The model under review builds one solid part; all positions refer to its coordinate system, in mm. A direction names the side the tool comes from. Give positions to 0.01 mm unless a question says otherwise; leave off trailing zeros. Write each loop counter-clockwise with the first axis right and the second up, starting at its lowest first coordinate (ties: lowest second). Pieces come first, ordered by that corner, then holes. Notation, with made-up numbers: M -38,-15 L -4,-15 A21 ccw -4,16 Z; hole C -20.75,62.25 d1. An arc over 180 degrees is marked long. Write item = value, one per line. Start each with the question number.
```python
from build123d import *

# Parameters (mm, degrees)
SKETCH_1_W          = 15
SKETCH_1_H          = 15
SKETCH_1_W_2        = 12
SKETCH_1_H_2        = 12
EXTRUDE_1_DEPTH     = 600
SKETCH_2_R          = 2.25
CUT_EXTRUDE_1_DEPTH = 25
SKETCH_3_R          = 2.25
CUT_EXTRUDE_2_DEPTH = 25
SKETCH_4_R          = 5
CUT_EXTRUDE_3_DEPTH = 10
SKETCH_5_R          = 5
CUT_EXTRUDE_4_DEPTH = 10
SKETCH_6_R          = 2.7
CUT_EXTRUDE_5_DEPTH = 20
SKETCH_7_R          = 5
CUT_EXTRUDE_6_DEPTH = 3


with BuildPart() as part:
    # ｽｹｯﾁ1 → ﾎﾞｽ - 押し出し1 (new body)
    with BuildSketch(Plane.XY):
        Rectangle(SKETCH_1_W, SKETCH_1_H)
        Rectangle(SKETCH_1_W_2, SKETCH_1_H_2, mode=Mode.SUBTRACT)
    extrude(amount=EXTRUDE_1_DEPTH)

    # ｽｹｯﾁ2 → ｶｯﾄ - 押し出し1 (cut)
    with BuildSketch(Plane(origin=(7.5, 0, 0), x_dir=(0, 0, -1), z_dir=(1, 0, 0))):
        with Locations((-592.5, 0)):
            Circle(SKETCH_2_R)
        with Locations((-7.5, 0)):
            Circle(SKETCH_2_R)
        with Locations((-336.5, 0)):
            Circle(SKETCH_2_R)
        with Locations((-263.5, 0)):
            Circle(SKETCH_2_R)
    extrude(amount=-CUT_EXTRUDE_1_DEPTH, mode=Mode.SUBTRACT)

    # ｽｹｯﾁ3 → ｶｯﾄ - 押し出し2 (cut)
    with BuildSketch(Plane(origin=(0, 7.5, 0), x_dir=(1, 0, 0), z_dir=(0, 1, 0))):
        with Locations((0, -22.5)):
            Circle(SKETCH_3_R)
        with Locations((0, -577.5)):
            Circle(SKETCH_3_R)
        with Locations((0, -351.5)):
            Circle(SKETCH_3_R)
        with Locations((0, -248.5)):
            Circle(SKETCH_3_R)
    extrude(amount=-CUT_EXTRUDE_2_DEPTH, mode=Mode.SUBTRACT)

    # ｽｹｯﾁ4 → ｶｯﾄ - 押し出し3 (cut)
    with BuildSketch(Plane(origin=(0, 7.5, 0), x_dir=(1, 0, 0), z_dir=(0, 1, 0))):
        with Locations((0, -577.5)):
            Circle(SKETCH_4_R)
        with Locations((0, -351.5)):
            Circle(SKETCH_4_R)
        with Locations((0, -248.5)):
            Circle(SKETCH_4_R)
        with Locations((0, -22.5)):
            Circle(SKETCH_4_R)
    extrude(amount=-CUT_EXTRUDE_3_DEPTH, mode=Mode.SUBTRACT)

    # ｽｹｯﾁ5 → ｶｯﾄ - 押し出し4 (cut)
    with BuildSketch(Plane(origin=(7.5, 0, 0), x_dir=(0, 0, -1), z_dir=(1, 0, 0))):
        with Locations((-592.5, 0)):
            Circle(SKETCH_5_R)
        with Locations((-336.5, 0)):
            Circle(SKETCH_5_R)
        with Locations((-263.5, 0)):
            Circle(SKETCH_5_R)
        with Locations((-7.5, 0)):
            Circle(SKETCH_5_R)
    extrude(amount=-CUT_EXTRUDE_4_DEPTH, mode=Mode.SUBTRACT)

    # ｽｹｯﾁ6 → ｶｯﾄ - 押し出し5 (cut)
    with BuildSketch(Plane(origin=(7.5, 0, 0), x_dir=(0, 0, -1), z_dir=(1, 0, 0))):
        with Locations((-480, 0)):
            Circle(SKETCH_6_R)
        with Locations((-443, 0)):
            Circle(SKETCH_6_R)
        with Locations((-157, 0)):
            Circle(SKETCH_6_R)
        with Locations((-120, 0)):
            Circle(SKETCH_6_R)
    extrude(amount=-CUT_EXTRUDE_5_DEPTH, mode=Mode.SUBTRACT)

    # ｽｹｯﾁ7 → ｶｯﾄ - 押し出し6 (cut)
    with BuildSketch(Plane.ZY.offset(7.5)):
        with Locations((120, 0)):
            Circle(SKETCH_7_R)
        with Locations((157, 0)):
            Circle(SKETCH_7_R)
        with Locations((443, 0)):
            Circle(SKETCH_7_R)
        with Locations((480, 0)):
            Circle(SKETCH_7_R)
    extrude(amount=-CUT_EXTRUDE_6_DEPTH, mode=Mode.SUBTRACT)


solid = part.part
```
Item 1: For faces 4 (the cylindrical face through (6.76, -1.915, 587.881)), 5 (the cylindrical face through (-1.08, 6.76, 27.38)), 6 (the cylindrical face through (-6.76, 1.5, 447.77)), 7 (the flat face through (7.5, 0, 296)), 8 (the flat face through (0, -6, 296)), list the 3-axis set-ups (+Z, -Z, +X, -X, +Y, -Y) from which the entire face can be reached by the end or side of a thin tool; tool diameter is ignored.
Item 2: To check wall thickness, follow probe 1 along Z at (x, y) = (0, 6.6); probe 2 along X at (y, z) = (7, 351.5); probe 3 along Y at (x, z) = (4.5, 437). State the ranges of each line that lie inside material, in increasing order. Write a range as [from, to].
Item 3: We need section A-A, the plane z = 228. Write out the cut boundary in (x, y), and give its area (3 significant figures).
Item 4: Clearance check with flat-ended pins moving along their axes: P1, Ø4.5, axis at y = 0, z = 480, coming from the -X side; P2, Ø6, axis at y = 0, z = 336.5, coming from the +X side; P3, Ø6, axis at x = 0, z = 22.5, coming from the +Y side; P4, Ø7, axis at y = 0, z = 157, coming from the -X side. State where each tip first meets the part, or that it passes through.
Item 5: The part is to be moulded in two halves that separate along Z. For faces 1 (the cylindrical face through (6.76, 1.5, 331.73)), 2 (the flat face through (-6, 0, 296)), 3 (the flat face through (-7, 0, 600)), say which applies: released by +Z, released by -Z, zero draft, split by the parting line, or undercut.
Worked out:
q1.face_4 = +X
q1.face_5 = +Y
q1.face_6 = -X
q1.face_7 = +Z, -Z, +X, +Y, -Y
q1.face_8 = +Z, -Z
q2.probe_1 = [0, 17.5], [27.5, 243.5], [253.5, 346.5], [356.5, 572.5], [582.5, 600]
q2.probe_2 = [-7.5, -5], [5, 7.5]
q2.probe_3 = [-7.5, -6], [6, 7.5]
q3.outline = M -7.5,-7.5 L 7.5,-7.5 L 7.5,7.5 L -7.5,7.5 Z; hole M -6,-6 L 6,-6 L 6,6 L -6,6 Z
q3.area = 81.0 mm²
q4.P1 = through
q4.P2 = -6
q4.P3 = -6
q4.P4 = 6
q5.face_1 = undercut
q5.face_2 = zero draft
q5.face_3 = released by +Z
